The drawing under review shows one solid part. Ordinate dimensions are in mm from its lowest x, y, z. Round coordinates to 2 decimals unless told otherwise and drop trailing zeros. Order: outer loops, then holes, each group sorted by start corner. A loop starts at its lowest first (then second) coordinate and runs counter-clockwise, first axis right, second up. Notation, with made-up numbers: M 74.5,47.5 L 95.5,47.5 A16 cw 95.5,61.5 Z; hole C 61.25,-27.5 d11. An arc over 180 degrees is marked long. Answer as a JSON object with one key per item and string values. Group by question number.
1) Consider section B-B, the plane x = 762. Write out the cut boundary in (y, z).
2) Insertion check: pin 1 Ø20.5 at (y, z) = (255, 421) entering from +X; pin 2 Ø7.5 at (y, z) = (248.5, 467.5) entering from -X. Each pin has a flat end and moves straight along its axis. Give the tip position at first contact, or say it passes through.
3) Consider section A-A, the plane z = 47.5. Write out the cut boundary in (x, y), then the cut area to 3 significant figures.
4) To check wall thickness, follow line 1 (Y direction, x = 1214, z = 529); line 2 (Z direction, x = 1114, y = 1083). State the ranges of each line that lie inside material, in increasing order.
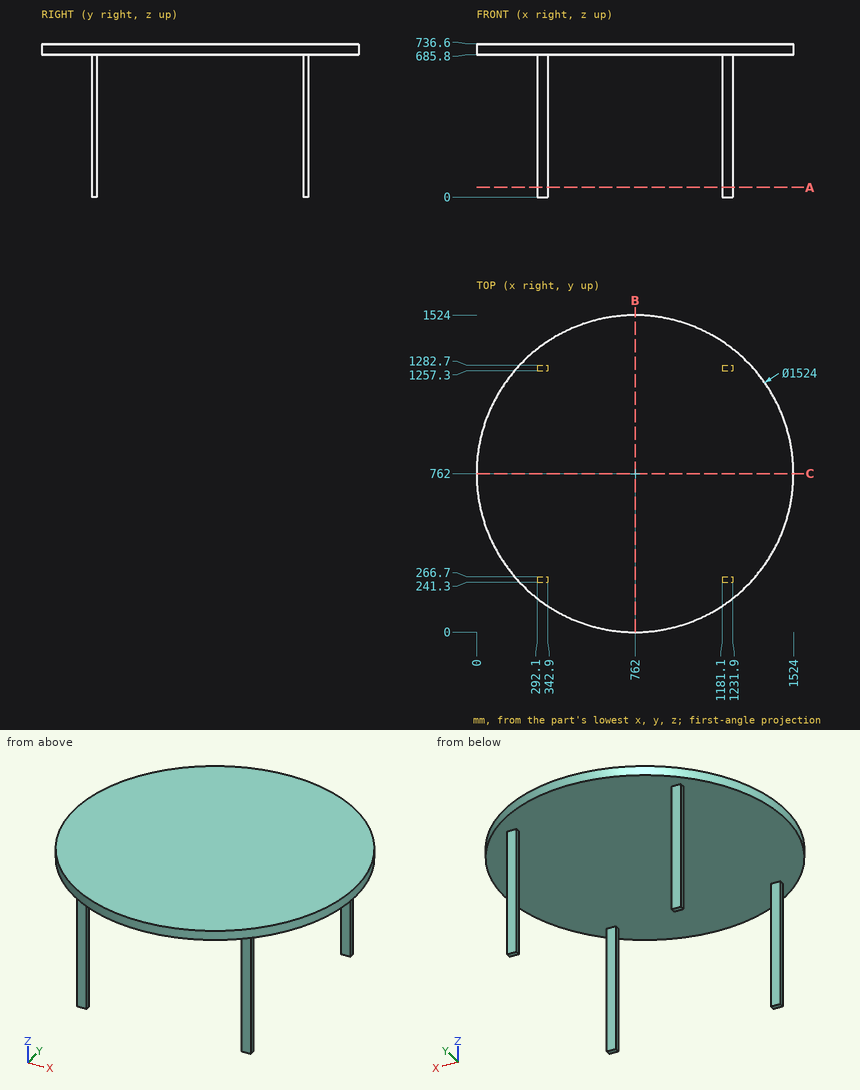
Results list:
{
 "1": {"outline": "M 0,685.8 L 1524,685.8 L 1524,736.6 L 0,736.6 Z"},
 "2": {"pin 1": "x = 1231.9", "pin 2": "x = 292.1"},
 "3": {"outline": "M 292.1,241.3 L 342.9,241.3 L 342.9,266.7 L 292.1,266.7 Z; M 292.1,1257.3 L 342.9,1257.3 L 342.9,1282.7 L 292.1,1282.7 Z; M 1181.1,241.3 L 1231.9,241.3 L 1231.9,266.7 L 1181.1,266.7 Z; M 1181.1,1257.3 L 1231.9,1257.3 L 1231.9,1282.7 L 1181.1,1282.7 Z", "area": "5,160 mm^2"},
 "4": {"line 1": "241.3 to 266.7, 1257.3 to 1282.7", "line 2": "685.8 to 736.6"}
}
